The model under review builds one solid part; all positions refer to its coordinate system, in mm. A direction names the side the tool comes from. Give positions to 0.01 mm unless a question says otherwise; leave off trailing zeros. Order: outer loops, then holes, each group sorted by start corner. A loop starts at its lowest first (then second) coordinate and runs counter-clockwise, first axis right, second up. Notation, with made-up numbers: M 89.25,6.5 L 132.25,6.5 A12 ccw 132.25,23.5 Z; hole C -1.5,37.25 d2. An arc over 180 degrees is marked long. One line per question, with ' | ' between items. Start each with the question number.
1. Wall thickness on L1, parallel to X at y = 0.9, z = -7 (3 decimals); L2, parallel to Z at x = -2, y = -0.75; L3, parallel to X at y = 1.4, z = -62: over which ranges is each line inside the solid? List them lowest first.
2. The part is to be moulded in two halves that separate along Z. For faces 1 (the face through (0.223, -0.019, 13.975)), 2 (the face through (0.346, 1.459, 34.796)), 3 (the face through (15.875, 0, -55)), 4 (the face through (-10.823, 1.459, -132.036)), say which applies: +Z half, -Z half, draft (parallel to the pull), parting line (faces both ways), or undercut.
3. For faces 5 (the face through (5.55, 0, -63)), 6 (the face through (-10.823, -1.462, -132.033)), list the 3-axis set-ups (+Z, -Z, +X, -X, +Y, -Y) from which the entire face can be reached by the end or side of a thin tool; tool diameter is ignored.
4. We need section A-A on y = 0.45. Write out the cut boundary in (x, z) (3 decimals).
```python
from build123d import *

# Parameters (mm, degrees)
SKETCH1_R          = 5.08
BASE_EXTRUDE_DEPTH = 1.5875
CHAMFER1_SIZE      = 0.254
EXTRUDE1_DEPTH     = 0.0254


with BuildPart() as part:
    # Sketch1 → Base-Extrude (new body, symmetric)
    with BuildSketch(Plane(origin=(0, 0, 0), x_dir=(1, 0, 0), z_dir=(0, 1, 0))):
        with BuildLine():
            Line((5.5499, 0), (5.5499, 127))
            ThreePointArc((5.5499, 127), (10.71245, 132.16255), (15.875, 127))
            Line((15.875, 127), (15.875, -19.05))
            ThreePointArc((15.875, -19.05), (0, -34.925), (-15.875, -19.05))
            Line((-15.875, -19.05), (-15.875, 127))
            ThreePointArc((-15.875, 127), (-10.71245, 132.16255), (-5.5499, 127))
            Line((-5.5499, 127), (-5.5499, 0))
            ThreePointArc((-5.5499, 0), (0, -5.5499), (5.5499, 0))
        make_face()
        with Locations(Location((0, -19.05, 0), (0, 0, 270))):  # turned: the seam where the file's is
            Circle(SKETCH1_R, mode=Mode.SUBTRACT)
    extrude(amount=BASE_EXTRUDE_DEPTH, both=True)

    # Chamfer1
    chamfer1_edges = [part.edges().sort_by_distance(p)[0] for p in [
        (-10.71245, 1.5875, -132.16255),
        (-5.5499, -1.5875, -63.5),
        (0, -1.5875, 5.5499),
        (-15.875, 1.5875, -53.975),
        (0, 1.5875, 34.925),
        (15.875, 1.5875, -53.975),
        (0, -1.5875, 13.97),
        (0, 1.5875, 13.97),
        (10.71245, 1.5875, -132.16255),
        (5.5499, 1.5875, -63.5),
        (0, 1.5875, 5.5499),
        (-5.5499, 1.5875, -63.5),
        (5.5499, -1.5875, -63.5),
        (10.71245, -1.5875, -132.16255),
        (15.875, -1.5875, -53.975),
        (0, -1.5875, 34.925),
        (-15.875, -1.5875, -53.975),
        (-10.71245, -1.5875, -132.16255),
    ]]
    chamfer(chamfer1_edges, length=CHAMFER1_SIZE)

    # Sketch2 → Extrude1 (cut)
    with BuildSketch(Plane(origin=(0, 1.5875, 0), x_dir=(1, 0, 0), z_dir=(0, 1, 0))):
        with BuildLine():
            add(Edge.make_bspline(
                [(-3.866987179, -30.058088124), (-3.849306773, -30.059138746), (-3.814646402, -30.061198369), (-3.764536622, -30.075328638), (-3.719184323, -30.100418994), (-3.678787215, -30.1338588), (-3.645489197, -30.174404152), (-3.619504678, -30.219394726), (-3.605497498, -30.269924028), (-3.603452878, -30.304785233), (-3.602403846, -30.322671457)],
                knots=[0, 0, 0, 0, 1.020151414, 1.999887582, 2.974338812, 3.990962822, 5.007586832, 5.987933904, 6.967670073, 8, 8, 8, 8], degree=3))
            add(Edge.make_bspline(
                [(-3.602403846, -30.322671457), (-3.603488427, -30.340127906), (-3.605627204, -30.374551768), (-3.61947257, -30.424699952), (-3.64568723, -30.469718643), (-3.678557545, -30.510814154), (-3.71919431, -30.544324801), (-3.764643842, -30.569201693), (-3.814528769, -30.584343703), (-3.849287148, -30.586272558), (-3.866987179, -30.58725479)],
                knots=[0, 0, 0, 0, 1.009421747, 1.99056486, 2.972319754, 3.999869655, 5.017953583, 5.993804169, 6.978383603, 8, 8, 8, 8], degree=3))
            add(Edge.make_bspline(
                [(-3.866987179, -30.58725479), (-3.884699965, -30.586308099), (-3.919279963, -30.584459908), (-3.968978686, -30.568890791), (-4.014705008, -30.544558081), (-4.055333861, -30.51075167), (-4.088479474, -30.469930112), (-4.113539643, -30.424389911), (-4.128589278, -30.374695321), (-4.130568548, -30.340156181), (-4.131570513, -30.322671457)],
                knots=[0, 0, 0, 0, 1.022052826, 1.995314843, 2.982371812, 4.00089066, 5.028879526, 6.005146991, 6.990147033, 8, 8, 8, 8], degree=3))
            add(Edge.make_bspline(
                [(-4.131570513, -30.322671457), (-4.130607037, -30.304755948), (-4.128725969, -30.269778116), (-4.113508049, -30.21970464), (-4.088673913, -30.174194699), (-4.055104734, -30.133920658), (-4.014714837, -30.100186463), (-3.969088993, -30.075634829), (-3.919160268, -30.061083883), (-3.884679823, -30.059104029), (-3.866987179, -30.058088124)],
                knots=[0, 0, 0, 0, 1.032775665, 2.016367738, 2.991239715, 4.008302682, 5.025365648, 6.011011707, 6.979408107, 8, 8, 8, 8], degree=3))
        make_face()
        Polygon((-2.520537861, -27.371549662), (-1.93349359, -27.371549662), (-1.93349359, -30.546549662), (-2.218429487, -30.546549662), (-2.218429487, -27.697190688), (-2.706891026, -27.697190688), align=None)
        Polygon((-0.691987179, -27.371549662), (-0.363166066, -27.371549662), (0.468108974, -28.670297659), (1.299384014, -27.371549662), (1.628205128, -27.371549662), (0.63283754, -28.927248781), (1.668910256, -30.546549662), (1.340089143, -30.546549662), (0.468108974, -29.184199903), (-0.403871194, -30.546549662), (-0.732692308, -30.546549662), (0.304016426, -28.927248781), align=None)
        Polygon((1.994551282, -27.371549662), (2.323372396, -27.371549662), (3.154647436, -28.670297659), (3.985922476, -27.371549662), (4.31474359, -27.371549662), (3.319376002, -28.927248781), (4.355448718, -30.546549662), (4.026627604, -30.546549662), (3.154647436, -29.184199903), (2.282667268, -30.546549662), (1.953846154, -30.546549662), (2.990554888, -28.927248781), align=None)
    extrude(amount=-EXTRUDE1_DEPTH, mode=Mode.SUBTRACT)


solid = part.part
```
Entries:
1) L1: x = -15.875 to -5.55, 5.55 to 15.875 | L2: z = 5.18 to 14.38, 23.72 to 34.8 | L3: x = -15.81 to -5.62, 5.62 to 15.81
2) face 1: undercut | face 2: +Z half | face 3: draft | face 4: -Z half
3) face 5: -Z, +Y, -Y | face 6: -Z, -Y
4) outline: M -15.875,-127 A5.163 ccw -5.55,-127 L -5.55,0 A5.55 cw 5.55,0 L 5.55,-127 A5.163 ccw 15.875,-127 L 15.875,19.05 A15.875 ccw -15.875,19.05 Z; hole C 0,19.05 d10.16
